Verification items for the finished model (mm, model axes). A direction names the side the tool comes from. Coordinates: 2 decimals unless noted, no trailing zeros. Loops run counter-clockwise (first coordinate to the right, second up) from the corner with the lowest first, then second, coordinate; pieces in that order, holes last. Notation, with made-up numbers: (3, 44.25) -> (23, 44.25) arc R12 ccw to (23, 63.25) -> close; hole circle Ø9 at (83.5, -8). An arc over 180 degrees is marked (long way). Answer as a JSON object with one key per item and string values. Group by question number.
Q1. Gauge pin test, flat ends, axial feed: pin 1 Ø5.5 at (x, z) = (-41.5, 46.5) entering from +Y; pin 2 Ø8 at (x, y) = (33.5, 5.5) entering from -Z; pin 3 Ø5.5 at (x, z) = (38.5, -43) entering from +Y; pin 4 Ø4 at (x, z) = (33.5, 36) entering from +Y. Record the tip position at first contact, or that the pin passes through.
Q2. Scan lines: L1, parallel to Z at x = -56, y = 2.75 (3 decimals); L2, parallel to X at y = 2.5, z = 49; L3, parallel to Z at x = -4.5, y = 7.25. Record each from-to range of solid material in increasing order.
Q3. Cross-section at A-A on x = -4. Record the boundary of the cut face in (y, z), and give its area (3 significant figures).
Q4. Cross-section at B-B on x = 45.5. Record the boundary of the cut face in (y, z).
Q5. Set-up check for faces 4 (the cylindrical face through (51.925, -0.478, -31.327)), 5 (the flat face through (43, -10, 38)), 6 (the flat face through (46.25, 1.66, -65.17)), 7 (the flat face through (23.17, 9, 53)), 8 (the flat face through (-52, 4.22, -28)): record each of +Z, -Z, +X, -X, +Y, -Y from which the full face is reachable in a straight line by a thin tool's end or side.
Q6. Release check for a two-part mould opening along Z. For faces 1 (the cylindrical face through (31.327, -0.478, 51.925)), 2 (the flat face through (28, -5.31, 55)), 3 (the flat face through (38, 11, -50.2)) record: released by +Z, released by -Z, zero draft, split by the parting line, or undercut.
```python
from build123d import *

# Parameters (mm, degrees)
SKETCH1_W                          = 139.7
SKETCH1_H                          = 139.7
BOSS_EXTRUDE1_DEPTH                = 12.7
POWER_SUPPLY_COMPONENT_DEPTH_DEPTH = 20.9
CUT_EXTRUDE6_DEPTH                 = 22.4
SKETCH8_W                          = 10.36
SKETCH8_H                          = 9.05
CUT_EXTRUDE7_DEPTH                 = 8.48
CUT_EXTRUDE8_DEPTH                 = 9.53
FILLET2_R                          = 2.2
CIRPATTERN5_COUNT                  = 4
FILLET2_OF_CIRPATTERN5_R           = 2.2
CUT_EXTRUDE9_DEPTH                 = 3.25
SKETCH12_W                         = 30
SKETCH12_H                         = 10
CUT_EXTRUDE10_DEPTH                = 101.969574625
FILLET5_R                          = 2
CIRPATTERN6_COUNT                  = 2
FILLET5_OF_CIRPATTERN6_R           = 2


with BuildPart() as part:
    # Sketch1 → Boss-Extrude1 (new, symmetric)
    with BuildSketch(Plane(origin=(0, 0, 0), x_dir=(1, 0, 0), z_dir=(0, 1, 0))):
        Rectangle(SKETCH1_W, SKETCH1_H)
    extrude(amount=BOSS_EXTRUDE1_DEPTH, both=True)

    # Sketch6 → power_supply_component_depth (cut)
    with BuildSketch(Plane(origin=(0, 12.7, 0), x_dir=(1, 0, 0), z_dir=(0, 1, 0))):
        with BuildLine():
            Line((-48, 39.868272016), (-48, -39.868272016))
            ThreePointArc((-48, -39.868272016), (-48, -48), (-39.868272016, -48))
            Line((-39.868272016, -48), (39.868272016, -48))
            ThreePointArc((39.868272016, -48), (48, -48), (48, -39.868272016))
            Line((48, -39.868272016), (48, 39.868272016))
            ThreePointArc((48, 39.868272016), (48, 48), (39.868272016, 48))
            Line((39.868272016, 48), (-39.868272016, 48))
            ThreePointArc((-39.868272016, 48), (-48, 48), (-48, 39.868272016))
        make_face()
    extrude(amount=-POWER_SUPPLY_COMPONENT_DEPTH_DEPTH, mode=Mode.SUBTRACT)

    # Sketch4 → Cut-Extrude6 (cut)
    with BuildSketch(Plane(origin=(0, 12.7, 0), x_dir=(1, 0, 0), z_dir=(0, 1, 0))):
        Polygon((-43.55, -69.85), (-50.940083446, -57.05), (-5.759916554, -57.05), (-13.15, -69.85), align=None)
        Polygon((43.55, -69.85), (36.159916554, -57.05), (20.540083446, -57.05), (13.15, -69.85), align=None)
    cut_extrude6 = extrude(amount=-CUT_EXTRUDE6_DEPTH, mode=Mode.SUBTRACT)

    # Sketch8 → Cut-Extrude7 (cut)
    with BuildSketch(Plane(origin=(0, 12.7, 0), x_dir=(1, 0, 0), z_dir=(0, 1, 0))):
        with Locations((-28.35, -52.525)):
            Rectangle(SKETCH8_W, SKETCH8_H)
        with Locations((28.35, -52.525)):
            Rectangle(SKETCH8_W, SKETCH8_H)
    cut_extrude7 = extrude(amount=-CUT_EXTRUDE7_DEPTH, mode=Mode.SUBTRACT)

    # Sketch9 → Cut-Extrude8 (cut)
    with BuildSketch(Plane(origin=(0, 4.22, 0), x_dir=(1, 0, 0), z_dir=(0, 1, 0))):
        with BuildLine():
            Line((27.085, -53.675), (29.615, -53.675))
            ThreePointArc((29.615, -53.675), (31.365, -51.925), (33.115, -53.675))
            Line((33.115, -53.675), (33.115, -57.05))
            Line((33.115, -57.05), (23.585, -57.05))
            Line((23.585, -57.05), (23.585, -53.675))
            ThreePointArc((23.585, -53.675), (25.335, -51.925), (27.085, -53.675))
        make_face()
    cut_extrude8 = extrude(amount=-CUT_EXTRUDE8_DEPTH, mode=Mode.SUBTRACT)

    # Fillet2
    fillet2_edges = [part.edges().sort_by_distance(p)[0] for p in [
        (-5.759916554, 1.5, 57.05),
        (-50.940083446, 1.5, 57.05),
        (36.159916554, 1.5, 57.05),
        (20.540083446, 1.5, 57.05),
    ]]
    fillet(fillet2_edges, radius=FILLET2_R)

    # CirPattern5: Cut-Extrude6, Cut-Extrude7, Cut-Extrude8 ×4 about axis
    cirpattern5_axis = Axis((0, 0, 0), (0, 1, 0))
    add([cut_extrude6.rotate(cirpattern5_axis, i * 360 / CIRPATTERN5_COUNT) for i in range(1, CIRPATTERN5_COUNT)], mode=Mode.SUBTRACT)
    add([cut_extrude7.rotate(cirpattern5_axis, i * 360 / CIRPATTERN5_COUNT) for i in range(1, CIRPATTERN5_COUNT)], mode=Mode.SUBTRACT)
    add([cut_extrude8.rotate(cirpattern5_axis, i * 360 / CIRPATTERN5_COUNT) for i in range(1, CIRPATTERN5_COUNT)], mode=Mode.SUBTRACT)

    # Fillet2 of CirPattern5
    fillet2_of_cirpattern5_edges = [part.edges().sort_by_distance(p)[0] for p in [
        (57.05, 1.5, 5.759916554),
        (57.05, 1.5, 50.940083446),
        (57.05, 1.5, -36.159916554),
        (57.05, 1.5, -20.540083446),
        (5.759916554, 1.5, -57.05),
        (50.940083446, 1.5, -57.05),
        (-36.159916554, 1.5, -57.05),
        (-20.540083446, 1.5, -57.05),
        (-57.05, 1.5, -5.759916554),
        (-57.05, 1.5, -50.940083446),
        (-57.05, 1.5, 36.159916554),
        (-57.05, 1.5, 20.540083446),
    ]]
    fillet(fillet2_of_cirpattern5_edges, radius=FILLET2_OF_CIRPATTERN5_R)

    # Sketch10 → Cut-Extrude9 (cut)
    with BuildSketch(Plane(origin=(0, 12.7, 0), x_dir=(1, 0, 0), z_dir=(0, 1, 0))):
        with BuildLine():
            Line((-42.068272016, 50.2), (42.068272016, 50.2))
            ThreePointArc((42.068272016, 50.2), (50.2, 50.2), (50.2, 42.068272016))
            Line((50.2, 42.068272016), (50.2, -42.068272016))
            ThreePointArc((50.2, -42.068272016), (50.2, -50.2), (42.068272016, -50.2))
            Line((42.068272016, -50.2), (-42.068272016, -50.2))
            ThreePointArc((-42.068272016, -50.2), (-50.2, -50.2), (-50.2, -42.068272016))
            Line((-50.2, -42.068272016), (-50.2, 42.068272016))
            ThreePointArc((-50.2, 42.068272016), (-50.2, 50.2), (-42.068272016, 50.2))
        make_face()
    extrude(amount=-CUT_EXTRUDE9_DEPTH, mode=Mode.SUBTRACT)

    # Sketch12 → Cut-Extrude10 (cut, symmetric)
    with BuildSketch(Plane(origin=(0, -8.2, 0), x_dir=(1, 0, 0), z_dir=(0, 1, 0))):
        with Locations((-28, 38)):
            Rectangle(SKETCH12_W, SKETCH12_H)
    cut_extrude10 = extrude(amount=CUT_EXTRUDE10_DEPTH, both=True, mode=Mode.SUBTRACT)

    # Fillet5
    fillet5_edges = [part.edges().sort_by_distance(p)[0] for p in [
        (-43, -10.45, -33),
        (-43, -10.45, -43),
        (-13, -10.45, -43),
        (-13, -10.45, -33),
    ]]
    fillet(fillet5_edges, radius=FILLET5_R)

    # CirPattern6: Cut-Extrude10 ×2 about axis
    cirpattern6_axis = Axis((0, 0, 0), (0, 1, 0))
    for i in range(1, CIRPATTERN6_COUNT):
        add(cut_extrude10.rotate(cirpattern6_axis, i * 360 / CIRPATTERN6_COUNT), mode=Mode.SUBTRACT)

    # Fillet5 of CirPattern6
    fillet5_of_cirpattern6_edges = [part.edges().sort_by_distance(p)[0] for p in [
        (43, -10.45, 33),
        (43, -10.45, 43),
        (13, -10.45, 43),
        (13, -10.45, 33),
    ]]
    fillet(fillet5_of_cirpattern6_edges, radius=FILLET5_OF_CIRPATTERN6_R)


solid = part.part
```
Computed values:
{
 "1": {"pin 1": "stops at y = 9.45", "pin 2": "stops at z = -57.05", "pin 3": "stops at y = -8.2", "pin 4": "passes through"},
 "2": {"L1": "z = -69.85 to 23.585, 33.115 to 69.85", "L2": "x = -69.85 to -46.65, -41.21 to 41.21, 46.65 to 58.09, 60.41 to 69.85", "L3": "z = -69.85 to -48, 48 to 69.85"},
 "3": {"outline": "(-12.7, -69.85) -> (12.7, -69.85) -> (12.7, -50.2) -> (9.45, -50.2) -> (9.45, -48) -> (-8.2, -48) -> (-8.2, 48) -> (9.45, 48) -> (9.45, 50.2) -> (12.7, 50.2) -> (12.7, 69.85) -> (-12.7, 69.85) -> close", "area": "1,530 mm²"},
 "4": {"outline": "(-12.7, -69.85) -> (12.7, -69.85) -> (12.7, -66.47) -> (-9.7, -66.47) -> (-9.7, -57.05) -> (12.7, -57.05) -> (12.7, -51.85) -> (9.45, -51.85) -> (9.45, -49.47) -> (-8.2, -49.47) -> (-8.2, 49.47) -> (9.45, 49.47) -> (9.45, 51.85) -> (12.7, 51.85) -> (12.7, 69.85) -> (-12.7, 69.85) -> close"},
 "5": {"face 4": "+X, +Y", "face 5": "+Y, -Y", "face 6": "+Y", "face 7": "+Z, -Z, +Y", "face 8": "+X, -X, +Y"},
 "6": {"face 1": "released by +Z", "face 2": "zero draft", "face 3": "undercut"}
}
